For this review, take the finished solid that the model builds, in its own axes (mm). Face numbers are marked on the shaded views. Round coordinates to 2 decimals unless told otherwise and drop trailing zeros. Write each loop counter-clockwise with the first axis right and the second up, starting at its lowest first coordinate (ties: lowest second). Pieces come first, ordered by that corner, then holes. Notation, with made-up numbers: (-35.5, -31.75) - (13.5, -31.75) arc R33 ccw to (13.5, -0.75) - close; hole circle Ø4 at (62.5, -1). An arc over 180 degrees is marked (long way). One line per item, written item: value. Start each with the question number.
Q1. Clearance check with flat-ended pins moving along their axes: pin 1 Ø13 at (x, z) = (-3, -4) entering from +Y; pin 2 Ø1.5 at (x, y) = (-14.5, 45.5) entering from -Z; pin 3 Ø8 at (x, y) = (7.5, 44) entering from +Z. State where each tip first meets the part, or that it passes through.
Q2. Add section B-B on z = 0. Write out the cut boundary in (x, y).
Q3. Add section A-A on x = 0. Write out the cut boundary in (y, z), and give its area (3 significant figures).
Q4. For probe 1 along Z at (x, y) = (-0.5, 49); probe 2 along Y at (x, z) = (-6, 13); probe 3 along X at (y, z) = (39, -5), list the stretches that pass through material, from the lowest coordinate up.
Q5. Mouldability with a two-part tool opening along Z and no side actions: class the marked faces 1, 2 and 3 as +Z half, -Z half, draft (parallel to the pull), parting line (faces both ways), or undercut.
Q6. Add section C-C on y = 16. Write out the cut boundary in (x, z), and give its area (3 significant figures).
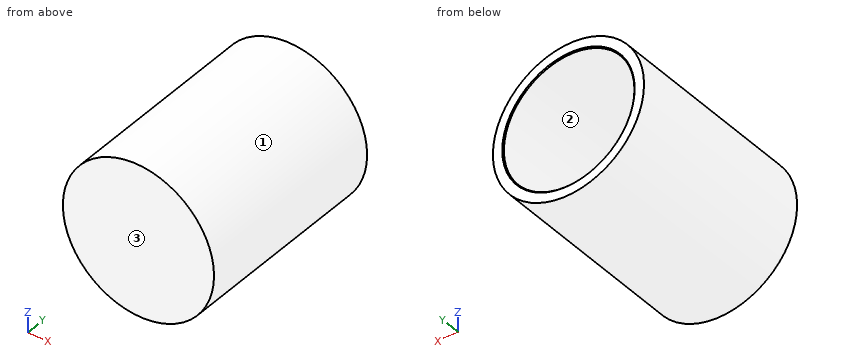
```python
from build123d import *

# Parameters (mm, degrees)
FILLET3_R     = 4
CHAMFER1_SIZE = 0.3569


with BuildPart() as part:
    # Main Revolve Sketch → Cylinder Main Revolve (revolve)
    with BuildSketch(Plane.XY, mode=Mode.PRIVATE) as cylinder_main_revolve_sk:
        Polygon((0, 0), (29.4, 0), (29.4, 77.4), (25.4, 77.4), (25.4, 4), (0, 4), align=None)
    revolve(cylinder_main_revolve_sk.sketch.rotate(Axis((0, 4, 0), (0, -1, 0)), 180), axis=Axis((0, 4, 0), (0, -1, 0)))

    # Fillet3
    fillet3_edges = [part.edges().sort_by_distance(p)[0] for p in [
        (25.4, 4, 0),
    ]]
    fillet(fillet3_edges, radius=FILLET3_R)

    # Chamfer1
    chamfer1_edges = [part.edges().sort_by_distance(p)[0] for p in [
        (25.4, 77.4, 0),
    ]]
    chamfer(chamfer1_edges, length=CHAMFER1_SIZE)


solid = part.part
```
Result set:
1. pin 1: stops at y = 4
1. pin 2: stops at z = -25.99
1. pin 3: stops at z = 29.19
2. outline: (-29.4, 0) - (29.4, 0) - (29.4, 77.4) - (25.76, 77.4) - (25.4, 77.04) - (25.4, 8) arc R4 cw to (21.4, 4) - (-21.4, 4) arc R4 cw to (-25.4, 8) - (-25.4, 77.04) - (-25.76, 77.4) - (-29.4, 77.4) - close
3. outline: (0, -29.4) - (77.4, -29.4) - (77.4, -25.76) - (77.04, -25.4) - (8, -25.4) arc R4 cw to (4, -21.4) - (4, 21.4) arc R4 cw to (8, 25.4) - (77.04, 25.4) - (77.4, 25.76) - (77.4, 29.4) - (0, 29.4) - close
3. area: 829 mm^2
4. probe 1: z = -29.4 to -25.4, 25.4 to 29.4
4. probe 2: y = 0 to 4
4. probe 3: x = -28.97 to -24.9, 24.9 to 28.97
5. face 1: parting line
5. face 2: undercut
5. face 3: draft
6. outline: circle Ø58.8 at (0, 0); hole circle Ø50.8 at (0, 0)
6. area: 689 mm^2
